Geometry: final body of the model. Coordinates: model frame, mm. A direction names the side the tool comes from. Coordinates: 2 decimals unless noted, no trailing zeros. Order: outer loops, then holes, each group sorted by start corner. A loop starts at its lowest first (then second) coordinate and runs counter-clockwise, first axis right, second up. Notation, with made-up numbers: M -24.5,0 L 29.5,0 A26 ccw 29.5,35 Z; hole C 30,27 d10. An arc over 180 degrees is marked long. One line per question, with ' | ' between items.
from build123d import *

# Parameters (mm, degrees)
SKETCH_W            = 104
SKETCH_H            = 34
PAD_DEPTH           = 9
SKETCH001_W         = 100
SKETCH001_H         = 32
POCKET_DEPTH        = 8
SKETCH002_R         = 2.5
SKETCH002_R_2       = 1.1
PAD001_DEPTH        = 2.5
SKETCH003_R         = 1.1
PAD002_DEPTH        = 4
SKETCH004_R         = 1.1
PAD003_DEPTH        = 4
SKETCH005_R         = 1.1
PAD004_DEPTH        = 4
SKETCH006_R         = 1.1
PAD005_DEPTH        = 4
POCKET001_DEPTH     = 1
SKETCH008_W         = 1
SKETCH008_H         = 32
PAD006_DEPTH        = 2
SKETCH009_W         = 1
SKETCH009_H         = 32
POCKET002_DEPTH     = 2
POCKET003_DEPTH     = 1
LINEARPATTERN_COUNT = 6
LINEARPATTERN_PITCH = 6
SKETCH011_W         = 3
SKETCH011_H         = 0.5
POCKET004_DEPTH     = 1
SKETCH012_W         = 3
SKETCH012_H         = 0.5
PAD007_DEPTH        = 1
SKETCH013_W         = 9
SKETCH013_H         = 0.5
POCKET005_DEPTH     = 1
SKETCH014_W         = 9
SKETCH014_H         = 0.5
PAD008_DEPTH        = 1
SKETCH015_R         = 0.5
POCKET006_DEPTH     = 1
SKETCH016_R         = 0.333333
PAD009_DEPTH        = 0.5
SKETCH017_W         = 3
SKETCH017_H         = 0.5
PAD010_DEPTH        = 1
SKETCH018_W         = 3
SKETCH018_H         = 0.5
POCKET007_DEPTH     = 1


with BuildPart() as part:
    # Sketch → Pad (new body)
    with BuildSketch(Plane.XY):
        with Locations((-52, 17)):
            Rectangle(SKETCH_W, SKETCH_H)
    extrude(amount=PAD_DEPTH)

    # Sketch001 (on Face6 of Pad) → Pocket (cut)
    with BuildSketch(Plane.XY.offset(9)):
        with Locations((-52, 17)):
            Rectangle(SKETCH001_W, SKETCH001_H)
    extrude(amount=-POCKET_DEPTH, mode=Mode.SUBTRACT)

    # Sketch002 (on Face11 of Pocket) → Pad001 (join)
    with BuildSketch(Plane.XY.offset(1)):
        with Locations((-65.5, 5.5)):
            Circle(SKETCH002_R)
        with Locations((-65.5, 28.7)):
            Circle(SKETCH002_R)
        with Locations((-7, 28.7)):
            Circle(SKETCH002_R)
        with Locations((-7, 5.5)):
            Circle(SKETCH002_R)
        with Locations((-17, 5.5)):
            Circle(SKETCH002_R_2)
    extrude(amount=PAD001_DEPTH)

    # Sketch003 (on Face17 of Pad001) → Pad002 (join)
    with BuildSketch(Plane.XY.offset(3.5)):
        with Locations((-7, 5.5)):
            Circle(SKETCH003_R)
    extrude(amount=PAD002_DEPTH)

    # Sketch004 (on Face20 of Pad002) → Pad003 (join)
    with BuildSketch(Plane.XY.offset(3.5)):
        with Locations((-7, 28.7)):
            Circle(SKETCH004_R)
    extrude(amount=PAD003_DEPTH)

    # Sketch005 (on Face21 of Pad003) → Pad004 (join)
    with BuildSketch(Plane.XY.offset(3.5)):
        with Locations((-65.5, 28.7)):
            Circle(SKETCH005_R)
    extrude(amount=PAD004_DEPTH)

    # Sketch006 (on Face19 of Pad004) → Pad005 (join)
    with BuildSketch(Plane.XY.offset(3.5)):
        with Locations((-65.5, 5.5)):
            Circle(SKETCH006_R)
    extrude(amount=PAD005_DEPTH)

    # Sketch007 (on Face6 of Pad005) → Pocket001 (cut)
    with BuildSketch(Plane.XZ):
        with BuildLine():
            ThreePointArc((-18, 8), (-19.5, 6.5), (-18, 5))
            Line((-18, 5), (-12, 5))
            ThreePointArc((-12, 5), (-10.5, 6.5), (-12, 8))
            Line((-18, 8), (-12, 8))
        make_face()
        with BuildLine():
            ThreePointArc((-30.5, 8), (-32, 6.5), (-30.5, 5))
            Line((-30.5, 5), (-24.5, 5))
            ThreePointArc((-24.5, 5), (-23, 6.5), (-24.5, 8))
            Line((-30.5, 8), (-24.5, 8))
        make_face()
    extrude(amount=-POCKET001_DEPTH, mode=Mode.SUBTRACT)

    # Sketch008 (on Face5 of Pocket001) → Pad006 (join)
    with BuildSketch(Plane.XY.offset(9)):
        with Locations((-102.5, 17)):
            Rectangle(SKETCH008_W, SKETCH008_H)
    extrude(amount=PAD006_DEPTH)

    # Sketch009 (on Face5 of Pad006) → Pocket002 (cut)
    with BuildSketch(Plane.XY.offset(9)):
        with Locations((-1.5, 17)):
            Rectangle(SKETCH009_W, SKETCH009_H)
    extrude(amount=-POCKET002_DEPTH, mode=Mode.SUBTRACT)

    # Sketch010 (on Face25 of Pocket002) → Pocket003 (cut)
    with BuildSketch(Plane.XY.offset(1)):
        with BuildLine():
            ThreePointArc((-65, 12), (-65.5, 11.5), (-65, 11))
            Line((-65, 11), (-62, 11))
            ThreePointArc((-62, 11), (-61.5, 11.5), (-62, 12))
            Line((-65, 12), (-62, 12))
        make_face()
        with BuildLine():
            ThreePointArc((-62, 14), (-62.5, 13.5), (-62, 13))
            Line((-62, 13), (-59, 13))
            ThreePointArc((-59, 13), (-58.5, 13.5), (-59, 14))
            Line((-62, 14), (-59, 14))
        make_face()
        with BuildLine():
            ThreePointArc((-65, 16), (-65.5, 15.5), (-65, 15))
            Line((-65, 15), (-62, 15))
            ThreePointArc((-62, 15), (-61.5, 15.5), (-62, 16))
            Line((-65, 16), (-62, 16))
        make_face()
    pocket003 = extrude(amount=-POCKET003_DEPTH, mode=Mode.SUBTRACT)

    # LinearPattern: Pocket003 ×6
    with Locations(*[(i * LINEARPATTERN_PITCH, 0, 0) for i in range(1, LINEARPATTERN_COUNT)]):
        add(pocket003, mode=Mode.SUBTRACT)

    # Sketch011 (on Face5 of LinearPattern) → Pocket004 (cut)
    with BuildSketch(Plane.XY.offset(9)):
        with Locations((-100.5, 33.25)):
            Rectangle(SKETCH011_W, SKETCH011_H)
        with Locations((-93.5, 33.25)):
            Rectangle(SKETCH011_W, SKETCH011_H)
        with Locations((-86.5, 33.25)):
            Rectangle(SKETCH011_W, SKETCH011_H)
        with Locations((-79.5, 33.25)):
            Rectangle(SKETCH011_W, SKETCH011_H)
    extrude(amount=-POCKET004_DEPTH, mode=Mode.SUBTRACT)

    # Sketch012 (on Face5 of Pocket004) → Pad007 (join)
    with BuildSketch(Plane.XY.offset(9)):
        with Locations((-3.5, 33.25)):
            Rectangle(SKETCH012_W, SKETCH012_H)
        with Locations((-10.5, 33.25)):
            Rectangle(SKETCH012_W, SKETCH012_H)
        with Locations((-17.5, 33.25)):
            Rectangle(SKETCH012_W, SKETCH012_H)
        with Locations((-24.5, 33.25)):
            Rectangle(SKETCH012_W, SKETCH012_H)
    extrude(amount=PAD007_DEPTH)

    # Sketch013 (on Face5 of Pad007) → Pocket005 (cut)
    with BuildSketch(Plane.XY.offset(9)):
        with Locations((-56.5, 0.75)):
            Rectangle(SKETCH013_W, SKETCH013_H)
    extrude(amount=-POCKET005_DEPTH, mode=Mode.SUBTRACT)

    # Sketch014 (on Face5 of Pocket005) → Pad008 (join)
    with BuildSketch(Plane.XY.offset(9)):
        with Locations((-47.5, 0.75)):
            Rectangle(SKETCH014_W, SKETCH014_H)
    extrude(amount=PAD008_DEPTH)

    # Sketch015 (on Face105 of Pad008) → Pocket006 (cut)
    with BuildSketch(Plane(origin=(-1, 0, 0), x_dir=(0, -1, 0), z_dir=(-1, 0, 0))):
        with Locations((-11.666667, 8)):
            Circle(SKETCH015_R)
        with Locations((-22.333333, 8)):
            Circle(SKETCH015_R)
    extrude(amount=-POCKET006_DEPTH, mode=Mode.SUBTRACT)

    # Sketch016 → Pad009 (join)
    with BuildSketch(Plane(origin=(-103, 0, 0), x_dir=(0, -1, 0), z_dir=(-1, 0, 0))):
        with Locations((-22.333333, 10)):
            Circle(SKETCH016_R)
        with Locations((-11.666667, 10)):
            Circle(SKETCH016_R)
    extrude(amount=PAD009_DEPTH)

    # Sketch017 (on Face5 of Pad009) → Pad010 (join)
    with BuildSketch(Plane.XY.offset(9)):
        with Locations((-3.5, 0.25)):
            Rectangle(SKETCH017_W, SKETCH017_H)
        with Locations((-10.5, 0.75)):
            Rectangle(SKETCH017_W, SKETCH017_H)
        with Locations((-17.5, 0.25)):
            Rectangle(SKETCH017_W, SKETCH017_H)
        with Locations((-24.5, 0.75)):
            Rectangle(SKETCH017_W, SKETCH017_H)
    extrude(amount=PAD010_DEPTH)

    # Sketch018 (on Face5 of Pad010) → Pocket007 (cut)
    with BuildSketch(Plane.XY.offset(9)):
        with Locations((-100.5, 0.25)):
            Rectangle(SKETCH018_W, SKETCH018_H)
        with Locations((-93.5, 0.75)):
            Rectangle(SKETCH018_W, SKETCH018_H)
        with Locations((-86.5, 0.25)):
            Rectangle(SKETCH018_W, SKETCH018_H)
        with Locations((-79.5, 0.75)):
            Rectangle(SKETCH018_W, SKETCH018_H)
    extrude(amount=-POCKET007_DEPTH, mode=Mode.SUBTRACT)


solid = part.part
1. Material intervals for line 1 (Y direction, x = -26.5, z = 1.25); line 2 (X direction, y = 26, z = 6.75); line 3 (X direction, y = 30.5, z = 8.25), sorted ascending. Write a range as [from, to].
Response values:
line 1: y = [0, 1], [33, 34] | line 2: x = [-104, -102], [-2, 0] | line 3: x = [-104, -102], [-1, 0]
2. Pin query (flat end, axial travel): P1, Ø0.6, axis at y = 0.5, z = 9.5, coming from the +X side. Return the tip coordinate at first contact, or that it passes through.
Response values:
P1: stops at x = -2
3. Section A-A, the plane x = -27. Output: boundary loops of the cut face in (y, z), and give its area (3 significant figures).
Response values:
outline: M 0,0 L 34,0 L 34,9 L 33,9 L 33,1 L 1,1 L 1,5 L 0,5 Z; M 0,8 L 1,8 L 1,9 L 0,9 Z | area: 47.0 mm^2
4. Access query for faces 5 (the face through (-5.85, 26.48, 2.23)), 6 (the face through (0, 17, 4)). Directions: +Z, -Z, +X, -X, +Y, -Y. A direction counts if a zero-diameter tool reaches every point of the face in a straight line with its end or side. Return the directions, or none.
Response values:
face 5: +Z | face 6: +Z, -Z, +X, +Y, -Y
5. Draft query along X for faces 1 (the face through (-52, 1, 4)), 2 (the face through (-7, 30, 3.5)), 3 (the face through (-104, 17, 4)), 4 (the face through (-53, 17, 0)). Return one class per face: pulls with the +X half, pulls with the -X half, needs draft (parallel to the pull), parting line crosses it, or undercut.
Response values:
face 1: undercut | face 2: undercut | face 3: pulls with the -X half | face 4: needs draft
6. Section B-B, the plane x = -89.5. Output: boundary loops of the cut face in (y, z).
Response values:
outline: M 0,0 L 34,0 L 34,9 L 33,9 L 33,1 L 1,1 L 1,9 L 0,9 Z
